from build123d import *

# Parameters (mm, degrees)
F0_W     = 52.938428
F0_H     = 19.312158
F0_W_2   = 46.482
F0_H_2   = 12.7
F1_DEPTH = 44.45
F2_W     = 46.482
F2_H     = 12.7
F3_DEPTH = 39.116
F4_R     = 1.905
F5_DEPTH = 58.674
F6_R     = 2.54


with BuildPart() as f1:
    # F0 (on Top) → F1 (new body)
    with BuildSketch(Plane.XY):
        Rectangle(F0_W, F0_H)
        Rectangle(F0_W_2, F0_H_2, mode=Mode.SUBTRACT)
        Rectangle(F0_W_2, F0_H_2)
    extrude(amount=F1_DEPTH)

    # F2 (on Top) → F3 (cut)
    with BuildSketch(Plane.XY):
        Rectangle(F2_W, F2_H)
    extrude(amount=F3_DEPTH, mode=Mode.SUBTRACT)

    # F4 (on Top) → F5 (cut)
    with BuildSketch(Plane.XY):
        Circle(F4_R)
    extrude(amount=F5_DEPTH, mode=Mode.SUBTRACT)

    # F6
    f6_edges = [f1.edges().sort_by_distance(p)[0] for p in [
        (-26.469214, 9.656079, 22.225),
        (26.469214, 9.656079, 22.225),
        (-26.469214, -9.656079, 22.225),
        (26.469214, -9.656079, 22.225),
    ]]
    fillet(f6_edges, radius=F6_R)


solid = f1.part
Design review of the part built by this model. Coordinates are the model's own, in mm. A direction names the side the tool comes from. Coordinates: 2 decimals unless noted, no trailing zeros. Loops run counter-clockwise (first coordinate to the right, second up) from the corner with the lowest first, then second, coordinate; pieces in that order, holes last. Notation, with made-up numbers: (82, 53) - (94, 53) arc R32 cw to (94, 84) - close; hole circle Ø11 at (-25.75, -7.75). An arc over 180 degrees is marked (long way). Use CSV: the item, a comma, the result in double quotes. Start each with the question number.
1. Add section A-A on z = 40.5. Give the boundary of the cut face in (x, y) (3 decimals), plus the area to 3 significant figures.
2. Add section C-C on x = 0. Give the boundary of the cut face in (y, z) (3 decimals), plus the area to 3 significant figures.
3. Add section B-B on y = 0. Give the boundary of the cut face in (x, z) (3 decimals), plus the area to 3 significant figures.
4. Clearance check with flat-ended pins moving along their axes: pin 1 (2.5 mm diameter, centred on x = 0, y = 0, fed in from -Z); pin 2 (3 mm diameter, centred on x = -13, y = 0.5, fed in from -Z). State where each tip first meets the part, or that it passes through.
5. Add section D-D on y = -5. Give the boundary of the cut face in (x, z).
6. To check wall thickness, follow probe 1 along Y at (x, z) = (-12, 21.5); probe 2 along Y at (x, z) = (0, 41.85) (3 decimals); probe 3 along X at (y, z) = (0.75, 31.5). State the ranges of each line that lie inside material, in increasing order.
7. For faces 1 (the flat face through (0, 6.35, 19)), 2 (the flat face through (-26.469, 0, 22)), list the 3-axis set-ups (+Z, -Z, +X, -X, +Y, -Y) from which the entire face can be reached by the end or side of a thin tool; tool diameter is ignored.
8. Mouldability with a two-part tool opening along Y and no side actions: class faces 3 (the cylindrical face through (-25.745, -8.892, 22.536)), 4 (the flat face through (0, 9.656, 22)), 5 (the flat face through (-0.4, 2.3, 44.45)), 6 (the flat face through (23.241, 0, 19)) as released by +Y, released by -Y, zero draft, split by the parting line, or undercut.
Resolved:
1,outline,"(-26.469, -7.116) arc R2.54 ccw to (-23.929, -9.656) - (23.929, -9.656) arc R2.54 ccw to (26.469, -7.116) - (26.469, 7.116) arc R2.54 ccw to (23.929, 9.656) - (-23.929, 9.656) arc R2.54 ccw to (-26.469, 7.116) - close; hole circle Ø3.81 at (0, 0)"
1,area,"1,010 mm2"
2,outline,"(-9.656, 0) - (-6.35, 0) - (-6.35, 39.116) - (-1.905, 39.116) - (-1.905, 44.45) - (-9.656, 44.45) - close; (1.905, 39.116) - (6.35, 39.116) - (6.35, 0) - (9.656, 0) - (9.656, 44.45) - (1.905, 44.45) - close"
2,area,"341 mm2"
3,outline,"(-26.469, 0) - (-23.241, 0) - (-23.241, 39.116) - (-1.905, 39.116) - (-1.905, 44.45) - (-26.469, 44.45) - close; (1.905, 39.116) - (23.241, 39.116) - (23.241, 0) - (26.469, 0) - (26.469, 44.45) - (1.905, 44.45) - close"
3,area,"515 mm2"
4,pin 1,"through"
4,pin 2,"z = 39.12"
5,outline,"(-26.47, 0) - (-23.24, 0) - (-23.24, 39.12) - (23.24, 39.12) - (23.24, 0) - (26.47, 0) - (26.47, 44.45) - (-26.47, 44.45) - close"
6,probe 1,"-9.66 to -6.35, 6.35 to 9.66"
6,probe 2,"-9.656 to -1.905, 1.905 to 9.656"
6,probe 3,"-26.47 to -23.24, 23.24 to 26.47"
7,face 1,"-Z"
7,face 2,"+Z, -Z, -X, +Y, -Y"
8,face 3,"released by -Y"
8,face 4,"released by +Y"
8,face 5,"zero draft"
8,face 6,"undercut"
